Here's how the part is built. I have some questions about the finished solid (model axes, mm). A direction names the side the tool comes from. Round coordinates to 2 decimals unless told otherwise and drop trailing zeros. Order: outer loops, then holes, each group sorted by start corner. A loop starts at its lowest first (then second) coordinate and runs counter-clockwise, first axis right, second up. Notation, with made-up numbers: (38, 60.25) - (42, 60.25) arc R21 cw to (42, 84.25) - close; hole circle Ø1 at (-3, 55). An arc over 180 degrees is marked (long way). Answer as a JSON object with one key per item and string values.
```python
from build123d import *

# Parameters (mm, degrees)
SKETCH1_R           = 5.1
BOSS_EXTRUDE1_DEPTH = 1
SKETCH2_R           = 4.3
SKETCH2_R_2         = 3.3
BOSS_EXTRUDE2_DEPTH = 2
SKETCH3_R           = 2.5
CUT_EXTRUDE1_DEPTH  = 2
SKETCH4_R           = 4.5
CUT_EXTRUDE2_DEPTH  = 0.5


with BuildPart() as part:
    # Sketch1 → Boss-Extrude1 (new body)
    with BuildSketch(Plane(origin=(0, 0, 0), x_dir=(1, 0, 0), z_dir=(0, 1, 0))):
        with Locations(Location((0, 0, 0), (0, 0, 270))):
            Circle(SKETCH1_R)
    extrude(amount=BOSS_EXTRUDE1_DEPTH)

    # Sketch2 → Boss-Extrude2 (add)
    with BuildSketch(Plane(origin=(0, 1, 0), x_dir=(1, 0, 0), z_dir=(0, 1, 0))):
        with Locations(Location((0, 0, 0), (0, 0, 270))):
            Circle(SKETCH2_R)
        with Locations(Location((0, 0, 0), (0, 0, 270))):
            Circle(SKETCH2_R_2, mode=Mode.SUBTRACT)
    extrude(amount=BOSS_EXTRUDE2_DEPTH)

    # Sketch3 → Cut-Extrude1 (cut)
    with BuildSketch(Plane.XZ):
        with Locations(Location((0, 0, 0), (0, 0, 270))):
            Circle(SKETCH3_R)
    extrude(amount=-CUT_EXTRUDE1_DEPTH, mode=Mode.SUBTRACT)

    # Sketch4 → Cut-Extrude2 (cut)
    with BuildSketch(Plane.XZ):
        with Locations(Location((0, 0, 0), (0, 0, 270))):
            Circle(SKETCH4_R)
    extrude(amount=-CUT_EXTRUDE2_DEPTH, mode=Mode.SUBTRACT)


solid = part.part
```
1. Imagine slicing it at D-D (x = 2.75). List the corners of the cut face in (y, z) for me, plus the area to 3 significant figures.
Responses:
{"outline": "(0, -4.3) - (1, -4.3) - (1, -3.31) - (3, -3.31) - (3, -1.82) - (1, -1.82) - (1, 1.82) - (3, 1.82) - (3, 3.31) - (1, 3.31) - (1, 4.3) - (0, 4.3) - (0, 3.56) - (0.5, 3.56) - (0.5, -3.56) - (0, -3.56) - close", "area": "11.0 mm2"}
2. For faces 1 (the face through (-2.44, 0.75, 0.54)), 2 (the face through (2, 1, -2)), 3 (the face through (-2, 0.5, -2)), which set-ups out of +Z, -Z, +X, -X, +Y, -Y let a thin tool reach every point of the face, with its end or its side?
Responses:
{"face 1": "+Y, -Y", "face 2": "+Y", "face 3": "-Y"}
3. For P1, Ø6, axis at x = 0, z = 0, coming from the -Y side; P2, Ø5, axis at x = 1.5, z = 0.5, coming from the +Y side; P3, Ø1, axis at y = 1, z = 2, coming from the +X side; P4, Ø6, axis at x = 0, z = 0, coming from the +Y side, each with a flat end and sliding along its axis, tell me the tip position at first contact or that it passes through.
Responses:
{"P1": "y = 0.5", "P2": "y = 3", "P3": "x = 4.87", "P4": "y = 1"}
4. Thinking about a two-plate mould opening in X: for faces 4 (the face through (-3, 3, 2)), 5 (the face through (1.532, 0.493, 4.864)), 6 (the face through (-2.008, 1.986, -2.619)), which applies, pulls with the +X half, pulls with the -X half, needs draft (parallel to the pull), parting line crosses it, or undercut?
Responses:
{"face 4": "needs draft", "face 5": "parting line crosses it", "face 6": "undercut"}
5. Imagine slicing it at B-B (x = -2.25). List the corners of the cut face in (y, z) for me.
Responses:
{"outline": "(0, -4.58) - (1, -4.58) - (1, -3.66) - (3, -3.66) - (3, -2.41) - (1, -2.41) - (1, -1.09) - (0.5, -1.09) - (0.5, -3.9) - (0, -3.9) - close; (0, 3.9) - (0.5, 3.9) - (0.5, 1.09) - (1, 1.09) - (1, 2.41) - (3, 2.41) - (3, 3.66) - (1, 3.66) - (1, 4.58) - (0, 4.58) - close"}
6. Imagine slicing it at A-A (z = 0). List the corners of the cut face in (x, y) for me, plus the area to 3 significant figures.
Responses:
{"outline": "(-5.1, 0) - (-4.5, 0) - (-4.5, 0.5) - (-2.5, 0.5) - (-2.5, 1) - (-3.3, 1) - (-3.3, 3) - (-4.3, 3) - (-4.3, 1) - (-5.1, 1) - close; (2.5, 0.5) - (4.5, 0.5) - (4.5, 0) - (5.1, 0) - (5.1, 1) - (4.3, 1) - (4.3, 3) - (3.3, 3) - (3.3, 1) - (2.5, 1) - close", "area": "7.20 mm2"}
7. Imagine slicing it at C-C (y = 1.7). List the corners of the cut face in (x, z) for me, plus the area to 3 significant figures.
Responses:
{"outline": "circle Ø8.6 at (0, 0); hole circle Ø6.6 at (0, 0)", "area": "23.9 mm2"}
8. If I drill on L1, parallel to X at y = 2.15, z = 0; L2, parallel to X at y = 0.25, z = 0; L3, parallel to Y at x = -1.75, z = -2.5, over which ranges is the centre line in solid material (lowest first)? Write a range as [from, to].
Responses:
{"L1": "[-4.3, -3.3], [3.3, 4.3]", "L2": "[-5.1, -4.5], [4.5, 5.1]", "L3": "[0.5, 1]"}
